from build123d import *

# Parameters (mm, degrees)
PLATES_DIMS_W                                    = 152.4
PLATES_DIMS_H                                    = 152.4
PLATE_THICKNESS_DEPTH                            = 9.525
F_4_40_TAPPED_HOLE1_D                            = 2.2606
LPATTERN1_COUNT                                  = 2
LPATTERN1_PITCH                                  = 139.7
LPATTERN1_COUNT_DIR2                             = 2
LPATTERN1_PITCH_DIR2                             = 139.7
LPATTERN3_COUNT                                  = 5
LPATTERN3_PITCH                                  = 25.4
LPATTERN4_COUNT                                  = 5
LPATTERN4_PITCH                                  = 25.4
BOTTOM_CONE_R                                    = 8.89
TOP_CONE_R                                       = 0.5
BOTTOM_GROOVE_W                                  = 17.78
BOTTOM_GROOVE_H                                  = 23.8125
TOP_GROOVE_W                                     = 1
TOP_GROOVE_H                                     = 23.8125
FLAT_DIMS_W                                      = 19.05
FLAT_DIMS_H                                      = 19.05
FLAT_CUT_LENGTH_DEPTH                            = 4.7112
F_1_4_20_TAPPED_HOLE2_D                          = 5.1054
CBORE_FOR_1_4_SOCKET_HEAD_CAP_SCREW1_D           = 6.7564
CBORE_FOR_1_4_SOCKET_HEAD_CAP_SCREW1_CBORE_D     = 11.1125
CBORE_FOR_1_4_SOCKET_HEAD_CAP_SCREW1_CBORE_DEPTH = 6.35
REST_TOP_CIRCLE_X_R                              = 7.5
REST_BOTTOM_CIRCLE_X_R                           = 0.5
REST_BOTTOM_CIRCLE_X_Z_R                         = 0.5
REST_TOP_CIRCLE_X_Z_R                            = 7.5
REST_BOTTOM_CIRCLE_X_Z_2_R                       = 0.5
REST_TOP_CIRCLE_X_Z_2_R                          = 7.5


with BuildPart() as part:
    # Plates_Dims → Plate_Thickness (new body)
    with BuildSketch(Plane(origin=(0, 0, 0), x_dir=(1, 0, 0), z_dir=(0, 1, 0))):
        Rectangle(PLATES_DIMS_W, PLATES_DIMS_H)
    extrude(amount=PLATE_THICKNESS_DEPTH)

    # #4-40 Tapped Hole1 (through all)
    with Locations(Plane(origin=(69.85, 9.525, 69.85), x_dir=(0, 0, 1), z_dir=(0, 1, 0))):
        with Locations((0, 0)):
            f_4_40_tapped_hole1 = Hole(F_4_40_TAPPED_HOLE1_D / 2)

    # LPattern1: 4-40 Tapped Hole1 2 × 2
    with Locations(*[(-j * LPATTERN1_PITCH_DIR2, 0, -i * LPATTERN1_PITCH) for i in range(LPATTERN1_COUNT) for j in range(LPATTERN1_COUNT_DIR2) if (i, j) != (0, 0)]):
        add(f_4_40_tapped_hole1, mode=Mode.SUBTRACT)

    # Sketch5 → #4-40 Tapped Hole3 (revolve, cut)
    with BuildSketch(Plane(origin=(-50.8, 4.7625, 76.2), x_dir=(0, -1, 0), z_dir=(1, 0, 0))):
        Polygon((0, 0), (0, 8.279152758), (1.1303, 7.6), (1.1303, 0), align=None)
    f_4_40_tapped_hole3 = revolve(axis=Axis((-50.8, 4.7625, 82.55), (0, 0, -1)), mode=Mode.SUBTRACT)

    # LPattern3: #4-40 Tapped Hole3 ×5
    with Locations(*[(i * LPATTERN3_PITCH, 0, 0) for i in range(1, LPATTERN3_COUNT)]):
        add(f_4_40_tapped_hole3, mode=Mode.SUBTRACT)

    # Sketch6 → #4-40 Tapped Hole4 (revolve, cut)
    with BuildSketch(Plane(origin=(-76.2, 4.7625, -50.8), x_dir=(0, 0, 1), z_dir=(0, 1, 0))):
        Polygon((0, 0), (0, 8.279152758), (1.1303, 7.6), (1.1303, 0), align=None)
    f_4_40_tapped_hole4 = revolve(axis=Axis((-82.55, 4.7625, -50.8), (1, 0, 0)), mode=Mode.SUBTRACT)

    # LPattern4: #4-40 Tapped Hole4 ×5
    with Locations(*[(0, 0, i * LPATTERN4_PITCH) for i in range(1, LPATTERN4_COUNT)]):
        add(f_4_40_tapped_hole4, mode=Mode.SUBTRACT)

    # Mirrior_Y: #4-40 Tapped Hole3 across plane
    add(f_4_40_tapped_hole3.mirror(Plane(origin=(0, 0, 0), x_dir=(1, 0, 0), z_dir=(0, 0, -1))), mode=Mode.SUBTRACT)

    # Mirrior_Y copy 1 sketch → Mirrior_Y copy 1 (revolve, cut)
    with BuildSketch(Plane(origin=(-25.4, 4.7625, -76.2), x_dir=(0, -1, 0), z_dir=(1, 0, 0))):
        Polygon((0, 0), (0, -8.279152758), (1.1303, -7.6), (1.1303, 0), align=None)
    revolve(axis=Axis((-25.4, 4.7625, -82.55), (0, 0, -1)), mode=Mode.SUBTRACT)

    # Mirrior_Y copy 2 sketch → Mirrior_Y copy 2 (revolve, cut)
    with BuildSketch(Plane(origin=(0, 4.7625, -76.2), x_dir=(0, -1, 0), z_dir=(1, 0, 0))):
        Polygon((0, 0), (0, -8.279152758), (1.1303, -7.6), (1.1303, 0), align=None)
    revolve(axis=Axis((0, 4.7625, -82.55), (0, 0, -1)), mode=Mode.SUBTRACT)

    # Mirrior_Y copy 3 sketch → Mirrior_Y copy 3 (revolve, cut)
    with BuildSketch(Plane(origin=(25.4, 4.7625, -76.2), x_dir=(0, -1, 0), z_dir=(1, 0, 0))):
        Polygon((0, 0), (0, -8.279152758), (1.1303, -7.6), (1.1303, 0), align=None)
    revolve(axis=Axis((25.4, 4.7625, -82.55), (0, 0, -1)), mode=Mode.SUBTRACT)

    # Mirrior_Y copy 4 sketch → Mirrior_Y copy 4 (revolve, cut)
    with BuildSketch(Plane(origin=(50.8, 4.7625, -76.2), x_dir=(0, -1, 0), z_dir=(1, 0, 0))):
        Polygon((0, 0), (0, -8.279152758), (1.1303, -7.6), (1.1303, 0), align=None)
    revolve(axis=Axis((50.8, 4.7625, -82.55), (0, 0, -1)), mode=Mode.SUBTRACT)

    # Mirror_X: #4-40 Tapped Hole4 across plane
    add(f_4_40_tapped_hole4.mirror(Plane.ZY), mode=Mode.SUBTRACT)

    # Mirror_X copy 1 sketch → Mirror_X copy 1 (revolve, cut)
    with BuildSketch(Plane(origin=(76.2, 4.7625, -25.4), x_dir=(0, 0, 1), z_dir=(0, 1, 0))):
        Polygon((0, 0), (0, -8.279152758), (1.1303, -7.6), (1.1303, 0), align=None)
    revolve(axis=Axis((82.55, 4.7625, -25.4), (1, 0, 0)), mode=Mode.SUBTRACT)

    # Mirror_X copy 2 sketch → Mirror_X copy 2 (revolve, cut)
    with BuildSketch(Plane(origin=(76.2, 4.7625, 0), x_dir=(0, 0, 1), z_dir=(0, 1, 0))):
        Polygon((0, 0), (0, -8.279152758), (1.1303, -7.6), (1.1303, 0), align=None)
    revolve(axis=Axis((82.55, 4.7625, 0), (1, 0, 0)), mode=Mode.SUBTRACT)

    # Mirror_X copy 3 sketch → Mirror_X copy 3 (revolve, cut)
    with BuildSketch(Plane(origin=(76.2, 4.7625, 25.4), x_dir=(0, 0, 1), z_dir=(0, 1, 0))):
        Polygon((0, 0), (0, -8.279152758), (1.1303, -7.6), (1.1303, 0), align=None)
    revolve(axis=Axis((82.55, 4.7625, 25.4), (1, 0, 0)), mode=Mode.SUBTRACT)

    # Mirror_X copy 4 sketch → Mirror_X copy 4 (revolve, cut)
    with BuildSketch(Plane(origin=(76.2, 4.7625, 50.8), x_dir=(0, 0, 1), z_dir=(0, 1, 0))):
        Polygon((0, 0), (0, -8.279152758), (1.1303, -7.6), (1.1303, 0), align=None)
    revolve(axis=Axis((82.55, 4.7625, 50.8), (1, 0, 0)), mode=Mode.SUBTRACT)

    # Bottom_Cone → Cone_Cut section 0
    with BuildSketch(Plane(origin=(0, 0, 0), x_dir=(1, 0, 0), z_dir=(0, 1, 0))):
        with Locations((-50.8, -50.8)):
            Circle(BOTTOM_CONE_R)
    # Top_Cone → Cone_Cut section 1
    with BuildSketch(Plane(origin=(0, 6.35, 0), x_dir=(-1, 0, 0), z_dir=(0, -1, 0))):
        with Locations((50.8, -50.8)):
            Circle(TOP_CONE_R)
    loft(mode=Mode.SUBTRACT)

    # Bottom_Groove → Groove_Cut section 0
    with BuildSketch(Plane(origin=(0, 0, 0), x_dir=(1, 0, 0), z_dir=(0, 1, 0))):
        with Locations((-50.8, 50.8)):
            Rectangle(BOTTOM_GROOVE_W, BOTTOM_GROOVE_H)
    # Top_Groove → Groove_Cut section 1
    with BuildSketch(Plane(origin=(0, 6.35, 0), x_dir=(-1, 0, 0), z_dir=(0, -1, 0))):
        with Locations((50.8, 50.8)):
            Rectangle(TOP_GROOVE_W, TOP_GROOVE_H)
    loft(mode=Mode.SUBTRACT)

    # Flat_Dims → Flat_Cut_Length (cut)
    with BuildSketch(Plane(origin=(0, 0, 0), x_dir=(1, 0, 0), z_dir=(0, 1, 0))):
        with Locations((50.8, 0)):
            Rectangle(FLAT_DIMS_W, FLAT_DIMS_H)
    extrude(amount=FLAT_CUT_LENGTH_DEPTH, mode=Mode.SUBTRACT)

    # 1/4-20 Tapped Hole2 (through all)
    with Locations(Plane(origin=(-31.75, 9.525, 0), x_dir=(0, 0, 1), z_dir=(0, 1, 0))):
        with Locations((0, 0), (0, 31.75), (31.75, 63.5), (-31.75, 63.5)):
            Hole(F_1_4_20_TAPPED_HOLE2_D / 2)

    # CBORE for 1/4 Socket Head Cap Screw1 (through all)
    with Locations(Plane(origin=(-50.8, 9.525, 0), x_dir=(0, 0, 1), z_dir=(0, 1, 0))):
        with Locations((0, 0), (50.8, 101.6), (-50.8, 101.6)):
            CounterBoreHole(CBORE_FOR_1_4_SOCKET_HEAD_CAP_SCREW1_D / 2, CBORE_FOR_1_4_SOCKET_HEAD_CAP_SCREW1_CBORE_D / 2, CBORE_FOR_1_4_SOCKET_HEAD_CAP_SCREW1_CBORE_DEPTH)

    # Rest_Top_Circle_X → Cut-Loft8 section 0
    with BuildSketch(Plane(origin=(0, 9.525, 0), x_dir=(1, 0, 0), z_dir=(0, 1, 0))):
        with Locations((31.75, 0)):
            Circle(REST_TOP_CIRCLE_X_R)
    # Rest_Bottom_Circle_X → Cut-Loft8 section 1
    with BuildSketch(Plane(origin=(0, 8.35, 0), x_dir=(-1, 0, 0), z_dir=(0, -1, 0))):
        with Locations((-31.75, 0)):
            Circle(REST_BOTTOM_CIRCLE_X_R)
    loft(mode=Mode.SUBTRACT)

    # Rest_Bottom_Circle_X-Z → Cut-Loft9 section 0
    with BuildSketch(Plane(origin=(0, 8.35, 0), x_dir=(-1, 0, 0), z_dir=(0, -1, 0))):
        with Locations((31.75, -31.75)):
            Circle(REST_BOTTOM_CIRCLE_X_Z_R)
    # Rest_Top_Circle_X-Z → Cut-Loft9 section 1
    with BuildSketch(Plane(origin=(0, 9.525, 0), x_dir=(1, 0, 0), z_dir=(0, 1, 0))):
        with Locations((-31.75, -31.75)):
            Circle(REST_TOP_CIRCLE_X_Z_R)
    loft(mode=Mode.SUBTRACT)

    # Rest_Bottom_Circle_X-Z 2 → Cut-Loft10 section 0
    with BuildSketch(Plane(origin=(0, 8.35, 0), x_dir=(-1, 0, 0), z_dir=(0, -1, 0))):
        with Locations((31.75, 31.75)):
            Circle(REST_BOTTOM_CIRCLE_X_Z_2_R)
    # Rest_Top_Circle_X-Z 2 → Cut-Loft10 section 1
    with BuildSketch(Plane(origin=(0, 9.525, 0), x_dir=(1, 0, 0), z_dir=(0, 1, 0))):
        with Locations((-31.75, 31.75)):
            Circle(REST_TOP_CIRCLE_X_Z_2_R)
    loft(mode=Mode.SUBTRACT)


solid = part.part
Read the model definition and answer for the solid it produces. Units are mm, in the model's axes. A direction names the side the tool comes from. Give positions to 0.01 mm unless a question says otherwise; leave off trailing zeros. One line per item, written item: value. Start each with the question number.
(1) A tool of negligible diameter and unlimited length cuts with its end or side. For faces 4 (the cylindrical face through (-54.1, 1.57, 0.73)), 5 (the flat face through (48, 3.175, -48)), 6 (the flat face through (60.325, 2, 0)), from which of +Z, -Z, +X, -X, +Y, -Y can it reach the whole face along a straight path? Write none if from no direction.
(2) Find the intervals of material crossed by line 1 (Z direction, x = 69.85, y = 3.25); line 2 (X direction, y = 0.5, z = 69.5); line 3 (X direction, y = 2.5, z = -5.5) (3 decimals), in increasing order.
(3) Determine the mould class of faces 1 (the flat face through (-76.2, 6, 1)), 2 (the flat face through (76.2, 6, 1)), 3 (the cylindrical face through (54.15, 1.57, -50.36)) for opening direction X: pulls with the +X half, pulls with the -X half, needs draft (parallel to the pull), parting line crosses it, or undercut.
(4) Flat-ended cylindrical pins translate along their axes: pin 1 Ø3 at (x, y) = (-50.8, 4.76) entering from +Z; pin 2 Ø0.5 at (x, z) = (-50.5, 51) entering from -Y; pin 3 Ø6 at (x, z) = (50.8, -50.8) entering from -Y; pin 4 Ø1.4 at (y, z) = (4.76, 50.8) entering from -X. Find the tip coordinate at first contact, or state that the pin passes through.
Results below:
1. face 4: +Y, -Y
1. face 5: +Y
1. face 6: -Y
2. line 1: z = -76.2 to -70.98, -68.72 to 68.72, 70.98 to 76.2
2. line 2: x = -76.2 to -70.92, -68.78 to 68.78, 70.92 to 76.2
2. line 3: x = -76.2 to 41.275, 60.325 to 76.2
3. face 1: pulls with the -X half
3. face 2: pulls with the +X half
3. face 3: undercut
4. pin 1: stops at z = 76.2
4. pin 2: stops at y = 6.27
4. pin 3: passes through
4. pin 4: stops at x = -68.34
